from build123d import *

# Parameters (mm, degrees)
SKETCH1_W           = 60.5
SKETCH1_H           = 47
BOSS_EXTRUDE1_DEPTH = 9.3
FILLET1_R           = 1.27
DRAFT1_ANGLE        = -1.5
FILLET2_R           = 0.635
SKETCH3_R           = 19
BOSS_EXTRUDE2_DEPTH = 24
SKETCH4_R           = 2
BOSS_EXTRUDE3_DEPTH = 4


with BuildPart() as part:
    # Sketch1 → Boss-Extrude1 (new body)
    with BuildSketch(Plane.XY):
        Rectangle(SKETCH1_W, SKETCH1_H)
    extrude(amount=BOSS_EXTRUDE1_DEPTH)

    # Fillet1
    fillet1_edges = [part.edges().sort_by_distance(p)[0] for p in [
        (30.25, -23.5, 4.65),
        (-30.25, -23.5, 4.65),
        (-30.25, 23.5, 4.65),
        (30.25, 23.5, 4.65),
    ]]
    fillet(fillet1_edges, radius=FILLET1_R)

    # Draft1
    draft1_faces = [part.faces().sort_by_distance(p)[0] for p in [
        (-29.878025612, -23.128025612, 4.65),
        (0, -23.5, 4.65),
        (29.878025612, -23.128025612, 4.65),
        (30.25, 0, 4.65),
        (29.878025612, 23.128025612, 4.65),
        (0, 23.5, 4.65),
        (-30.25, 0, 4.65),
        (-29.878025612, 23.128025612, 4.65),
    ]]
    draft(draft1_faces, Plane(origin=(0, 0, 0), x_dir=(-1, 0, 0), z_dir=(0, 0, -1)), DRAFT1_ANGLE)

    # Fillet2
    fillet2_edges = [part.edges().sort_by_distance(p)[0] for p in [
        (0, -23.256470929, 9.3),
        (-30.006470929, 0, 9.3),
        (30.006470929, 0, 9.3),
        (0, 23.256470929, 9.3),
        (-29.705824555, 22.955824555, 9.3),
        (29.705824555, 22.955824555, 9.3),
        (29.705824555, -22.955824555, 9.3),
        (-29.705824555, -22.955824555, 9.3),
    ]]
    fillet(fillet2_edges, radius=FILLET2_R)

    # Sketch3 → Boss-Extrude2 (add)
    with BuildSketch(Plane(origin=(0, 0, 0), x_dir=(-1, 0, 0), z_dir=(0, 0, -1))):
        Circle(SKETCH3_R)
    extrude(amount=BOSS_EXTRUDE2_DEPTH)

    # Sketch4 → Boss-Extrude3 (add)
    with BuildSketch(Plane(origin=(0, 0, -24), x_dir=(-1, 0, 0), z_dir=(0, 0, -1))):
        Circle(SKETCH4_R)
    extrude(amount=BOSS_EXTRUDE3_DEPTH)


solid = part.part
Source: CAD feature listing. Evaluate the final solid. Frame: model axes, mm. A direction names the side the tool comes from. Give positions to 0.01 mm unless a question says otherwise; leave off trailing zeros. Loops run counter-clockwise (first coordinate to the right, second up) from the corner with the lowest first, then second, coordinate; pieces in that order, holes last. Notation, with made-up numbers: (74, -21.75) -> (115, -21.75) arc R14 ccw to (115, -14.75) -> close; hole circle Ø7 at (9, -2.5). An arc over 180 degrees is marked (long way). Use a Markdown table: item, result. Add a question column.
1) Section query D-D, the plane x = 24. Return the cut outline in (y, z) (3 decimals), then the cut area to 3 significant figures.
2) Section query C-C, the plane z = -9.5. Return the cut outline in (x, y).
3) Pull-direction query (Z, two-part tool) for faces 1 (the face through (20, 0, 0)), 2 (the face through (0, 0, 9.3)), 3 (the face through (0, -2, -26)); classes: +Z half, -Z half, draft (parallel to the pull), parting line (faces both ways), or undercut.
4) Reachability of faces 4 (the face through (0, 0, -28)), 5 (the face through (-8.767, -16.856, -11.832)) from +Z, -Z, +X, -X, +Y, -Y: full face, straight path, thin tool, end or side. Return the list, or none.
5) Section query A-A, the plane x = 0. Return the cut outline in (y, z) (3 decimals), then the cut area to 3 significant figures.
6) First-contact query: pin 1 (2 mm diameter, centred on x = 10, z = -22.5, fed in from +Y); pin 2 (1 mm diameter, centred on y = 2, z = -9.5, fed in from -X); pin 3 (8 mm diameter, centred on x = -12, z = -16, fed in from -Y). Flat tips, straight axial feed; report the tip coordinate or a pass-through.
7) Line query: line 1 along Z through (x, y) = (5, 16); line 2 along Z through (x, y) = (-7.5, -19); line 3 along X through (y, z) = (19, 0.5). Output: solid intervals per line, ascending. Write a range as [from, to].
8) Section query B-B, the plane y = 0. Return the cut outline in (x, z) (3 decimals).
Numbers:
| question | item | result |
|---|---|---|
| 1 | outline | (-23.5, 0) -> (23.5, 0) -> (23.273, 8.682) arc R0.635 ccw to (22.638, 9.3) -> (-22.638, 9.3) arc R0.635 ccw to (-23.273, 8.682) -> close |
| 1 | area | 435 mm2 |
| 2 | outline | circle Ø38 at (0, 0) |
| 3 | face 1 | -Z half |
| 3 | face 2 | +Z half |
| 3 | face 3 | draft |
| 4 | face 4 | -Z, +X, -X, +Y, -Y |
| 4 | face 5 | -Z |
| 5 | outline | (-23.5, 0) -> (-19, 0) -> (-19, -24) -> (-2, -24) -> (-2, -28) -> (2, -28) -> (2, -24) -> (19, -24) -> (19, 0) -> (23.5, 0) -> (23.273, 8.682) arc R0.635 ccw to (22.638, 9.3) -> (-22.638, 9.3) arc R0.635 ccw to (-23.273, 8.682) -> close |
| 5 | area | 1,360 mm2 |
| 6 | pin 1 | stops at y = 16.73 |
| 6 | pin 2 | stops at x = -18.94 |
| 6 | pin 3 | stops at y = -17.23 |
| 7 | line 1 | z = [-24, 9.3] |
| 7 | line 2 | z = [0, 9.3] |
| 7 | line 3 | x = [-30.24, 30.24] |
| 8 | outline | (-30.25, 0) -> (-19, 0) -> (-19, -24) -> (-2, -24) -> (-2, -28) -> (2, -28) -> (2, -24) -> (19, -24) -> (19, 0) -> (30.25, 0) -> (30.023, 8.682) arc R0.635 ccw to (29.388, 9.3) -> (-29.388, 9.3) arc R0.635 ccw to (-30.023, 8.682) -> close |
